```python
from build123d import *

# Parameters (mm, degrees)
SKETCH1_W                                      = 40
SKETCH1_H                                      = 42
BOSS_EXTRUDE1_DEPTH                            = 2.5
SKETCH2_W                                      = 40
SKETCH2_H                                      = 2.5
BOSS_EXTRUDE2_DEPTH                            = 12
SKETCH3_R                                      = 1.75
BOSS_EXTRUDE3_DEPTH                            = 1.5
SKETCH5_R                                      = 0.89
CUT_EXTRUDE2_DEPTH                             = 31.842341027
SKETCH6_W                                      = 10
SKETCH6_H                                      = 5
CUT_EXTRUDE3_DEPTH                             = 31.842341027
CSK_FOR_M3_FLAT_HEAD_MACHINE_SCREW1_AT_2_COUNT = 2
CSK_FOR_M3_FLAT_HEAD_MACHINE_SCREW1_AT_2_PITCH = 30
BOSS_EXTRUDE4_DEPTH                            = 2.5
BOSS_EXTRUDE5_DEPTH                            = 39.5
BODY_MOVE_COPY1_ANGLE                          = 90


with BuildPart() as part:
    # Sketch1 → Boss-Extrude1 (new body)
    with BuildSketch(Plane(origin=(0, 0, 0), x_dir=(1, 0, 0), z_dir=(0, 1, 0))):
        Rectangle(SKETCH1_W, SKETCH1_H)
    extrude(amount=BOSS_EXTRUDE1_DEPTH)

    # Sketch2 → Boss-Extrude2 (add)
    with BuildSketch(Plane(origin=(0, 2.5, 0), x_dir=(1, 0, 0), z_dir=(0, 1, 0))):
        with Locations((0, 19.75)):
            Rectangle(SKETCH2_W, SKETCH2_H)
    extrude(amount=BOSS_EXTRUDE2_DEPTH)

    # Sketch3 → Boss-Extrude3 (add)
    with BuildSketch(Plane(origin=(0, 2.5, 0), x_dir=(1, 0, 0), z_dir=(0, 1, 0))):
        with Locations(Location((14, 13, 0), (0, 0, 90))):
            Circle(SKETCH3_R)
        with Locations(Location((-14, 13, 0), (0, 0, 90))):
            Circle(SKETCH3_R)
        with Locations(Location((-14, -15, 0), (0, 0, 90))):
            Circle(SKETCH3_R)
        with Locations(Location((14, -15, 0), (0, 0, 90))):
            Circle(SKETCH3_R)
    extrude(amount=BOSS_EXTRUDE3_DEPTH)

    # Sketch5 → Cut-Extrude2 (cut, through all)
    with BuildSketch(Plane(origin=(0, 4, 0), x_dir=(1, 0, 0), z_dir=(0, 1, 0))):
        with Locations(Location((-14, 13, 0), (0, 0, 270))):
            Circle(SKETCH5_R)
        with Locations(Location((14, 13, 0), (0, 0, 270))):
            Circle(SKETCH5_R)
        with Locations(Location((14, -15, 0), (0, 0, 270))):
            Circle(SKETCH5_R)
        with Locations(Location((-14, -15, 0), (0, 0, 270))):
            Circle(SKETCH5_R)
    extrude(amount=-CUT_EXTRUDE2_DEPTH, mode=Mode.SUBTRACT)

    # Sketch6 → Cut-Extrude3 (cut, through all)
    with BuildSketch(Plane(origin=(0, 4, 0), x_dir=(1, 0, 0), z_dir=(0, 1, 0))):
        with Locations((7.25, 13)):
            Rectangle(SKETCH6_W, SKETCH6_H)
    extrude(amount=-CUT_EXTRUDE3_DEPTH, mode=Mode.SUBTRACT)

    # Sketch8 → CSK for M3 Flat Head Machine Screw1 (revolve, cut)
    with BuildSketch(Plane(origin=(-15, 10.59833188, -18.5), x_dir=(0, -1, 0), z_dir=(1, 0, 0))):
        Polygon((0, 0), (0, 2.5), (1.7, 2.5), (1.7, 1.45), (3.15, 0), align=None)
    csk_for_m3_flat_head_machine_screw1 = revolve(axis=Axis((-15, 10.59833188, -12.15), (0, 0, -1)), mode=Mode.SUBTRACT)

    # CSK for M3 Flat Head Machine Screw1 at 2: CSK for M3 Flat Head Machine Screw1 ×2
    with Locations(*[Vector(0.9999946282308037, -0.0032777293263655718, 0) * (i * CSK_FOR_M3_FLAT_HEAD_MACHINE_SCREW1_AT_2_PITCH) for i in range(1, CSK_FOR_M3_FLAT_HEAD_MACHINE_SCREW1_AT_2_COUNT)]):
        add(csk_for_m3_flat_head_machine_screw1, mode=Mode.SUBTRACT)

    # Sketch9 → Boss-Extrude4 (add)
    with BuildSketch(Plane(origin=(0, 0, -21), x_dir=(-1, 0, 0), z_dir=(0, 0, -1))):
        Polygon((20, 0), (34.5, 14.5), (20, 14.5), align=None)
        Polygon((-20, 0), (-34.5, 14.5), (-20, 14.5), align=None)
    extrude(amount=-BOSS_EXTRUDE4_DEPTH)

    # Sketch10 → Boss-Extrude5 (add)
    with BuildSketch(Plane.XY.offset(-18.5)):
        Polygon((20, 2.5), (32, 14.5), (34.5, 14.5), (20, 0), align=None)
        Polygon((-20, 2.5), (-32, 14.5), (-34.5, 14.5), (-20, 0), align=None)
    extrude(amount=BOSS_EXTRUDE5_DEPTH)


with BuildPart() as part_1:
    # Body-Move/Copy1: moved
    add(part.part.rotate(Axis((0, 0, 0), (1, 0, 0)), BODY_MOVE_COPY1_ANGLE))


solid = part_1.part
```
Could you check a few things on this model? Use its own coordinates, in mm. A direction names the side the tool comes from. Give positions to 0.01 mm unless a question says otherwise; leave off trailing zeros. Loops run counter-clockwise (first coordinate to the right, second up) from the corner with the lowest first, then second, coordinate; pieces in that order, holes last. Notation, with made-up numbers: (-31, -7.5) -> (26, -7.5) arc R22 ccw to (26, 11.5) -> close; hole circle Ø6 at (26, 28). An arc over 180 degrees is marked (long way). Put each result on its own line as item: value.
(1) For faces 1 (the face through (12.5, 13.9, 3.2)), 2 (the face through (15, 14, 4)), 3 (the face through (0, 0, 0)), 4 (the face through (27, 0, 7)), 5 (the face through (7, 15.5, 1)), which set-ups out of +Z, -Z, +X, -X, +Y, -Y let a thin tool reach every point of the face, with its end or its side?
Computed:
face 1: +Z
face 2: +Z, -Y
face 3: -Z, +X, -X, +Y, -Y
face 4: -Z, +X, +Y, -Y
face 5: +Z, -Z
(2) I'm going to push flat-ended pins straight in: pin 1 Ø2 at (y, z) = (12.5, 1) entering from +X; pin 2 Ø5 at (x, z) = (-13, 5.5) entering from -Y; pin 3 Ø2 at (x, z) = (15, 10.5) entering from +Y; pin 4 Ø2 at (x, y) = (14, -15) entering from +Z. Where does each tip first touch, or does it pass through?
Computed:
pin 1: x = 22
pin 2: y = -16.75
pin 3: through
pin 4: z = 4
(3) Imagine slicing it at A-A on y = -15. Write out the boundary of the cut face in (x, z), plus the area to 3 significant figures.
Computed:
outline: (-34.5, 14.5) -> (-20, 0) -> (-14.89, 0) -> (-14.89, 4) -> (-15.75, 4) -> (-15.75, 2.5) -> (-20, 2.5) -> (-32, 14.5) -> close; (-13.11, 0) -> (13.11, 0) -> (13.11, 4) -> (12.25, 4) -> (12.25, 2.5) -> (-12.25, 2.5) -> (-12.25, 4) -> (-13.11, 4) -> close; (14.89, 0) -> (20, 0) -> (34.5, 14.5) -> (32, 14.5) -> (20, 2.5) -> (15.75, 2.5) -> (15.75, 4) -> (14.89, 4) -> close
area: 163 mm^2
(4) Imagine slicing it at C-C on z = 6.5. Write out the boundary of the cut face in (x, y), plus the area to 3 significant figures.
Computed:
outline: (-26.5, -21) -> (-24, -21) -> (-24, 18.5) -> (24, 18.5) -> (24, -21) -> (26.5, -21) -> (26.5, 21) -> (-26.5, 21) -> close
area: 330 mm^2
(5) Imagine slicing it at D-D on y = 6.5. Write out the boundary of the cut face in (x, z), plus the area to 3 significant figures.
Computed:
outline: (-34.5, 14.5) -> (-20, 0) -> (20, 0) -> (34.5, 14.5) -> (32, 14.5) -> (20, 2.5) -> (-20, 2.5) -> (-32, 14.5) -> close
area: 166 mm^2
(6) Imagine slicing it at B-B on x = 10. Write out the boundary of the cut face in (y, z).
Computed:
outline: (-21, 0) -> (10.5, 0) -> (10.5, 2.5) -> (-21, 2.5) -> close; (15.5, 0) -> (21, 0) -> (21, 14.5) -> (18.5, 14.5) -> (18.5, 2.5) -> (15.5, 2.5) -> close
(7) Thinking about a two-plate mould opening in Z: for faces 6 (the face through (-13.96, -14.11, 2.03)), 7 (the face through (16.5, 20.5, 9.7)), 8 (the face through (-27, 0, 7)), 9 (the face through (0, -1, 2.5)), which applies, pulls with the +Z half, pulls with the -Z half, needs draft (parallel to the pull), parting line crosses it, or undercut?
Computed:
face 6: needs draft
face 7: undercut
face 8: pulls with the -Z half
face 9: pulls with the +Z half
(8) Please list where these lines run through material, in increasing order: probe 1 along Z at (x, y) = (-15, 20.5); probe 2 along X at (y, z) = (13, 2.15); probe 3 along X at (y, z) = (-15, 2.1). Write a range as [from, to].
Computed:
probe 1: [0, 8.9], [12.3, 14.5]
probe 2: [-22.15, -14.89], [-13.11, 2.25], [12.25, 13.11], [14.89, 22.15]
probe 3: [-22.1, -14.89], [-13.11, 13.11], [14.89, 22.1]
